Input: part model. Units: mm. Frame: model coordinates. Coordinates: 2 decimals unless noted, no trailing zeros. Order: outer loops, then holes, each group sorted by start corner. A loop starts at its lowest first (then second) coordinate and runs counter-clockwise, first axis right, second up. Notation, with made-up numbers: (-26, 75) - (-21, 75) arc R12 cw to (-21, 88) - close; hole circle Ø8 at (-11.75, 68). An arc over 180 degrees is marked (long way). Use a Markdown table: item, result. Add a question column.
from build123d import *

# Parameters (mm, degrees)
SKETCH1_R           = 9.486832981
BOSS_EXTRUDE1_DEPTH = 11
FILLET1_R           = 0.5


with BuildPart() as part:
    # Sketch1 → Boss-Extrude1 (new body)
    with BuildSketch(Plane(origin=(0, 0, 0), x_dir=(1, 0, 0), z_dir=(0, 1, 0))):
        with Locations(Location((0, 0, 0), (0, 0, 270))):
            Circle(SKETCH1_R)
    boss_extrude1 = extrude(amount=BOSS_EXTRUDE1_DEPTH)

    # Sketch2 → Revolve1 (revolve)
    with BuildSketch(Plane.XY):
        with BuildLine():
            Line((0, 24.281566173), (0, 11))
            Line((0, 11), (-15.178932769, 11))
            add(Edge.make_bspline(
                [(0, 24.281566173), (-13.015575695, 23.967255227), (-15.178932769, 11)],
                knots=[0, 0, 0, 1, 1, 1], degree=2))
        make_face()
    revolve1 = revolve(axis=Axis((0, 0, 0), (0, 1, 0)))

    # Mirror1: Boss-Extrude1, Revolve1 across plane
    add(boss_extrude1.mirror(Plane.ZX))
    add(revolve1.mirror(Plane.ZX))

    # Fillet1
    fillet1_edges = [part.edges().sort_by_distance(p)[0] for p in [
        (0, -11, -9.486832981),
        (0, 11, -9.486832981),
    ]]
    fillet(fillet1_edges, radius=FILLET1_R)


solid = part.part
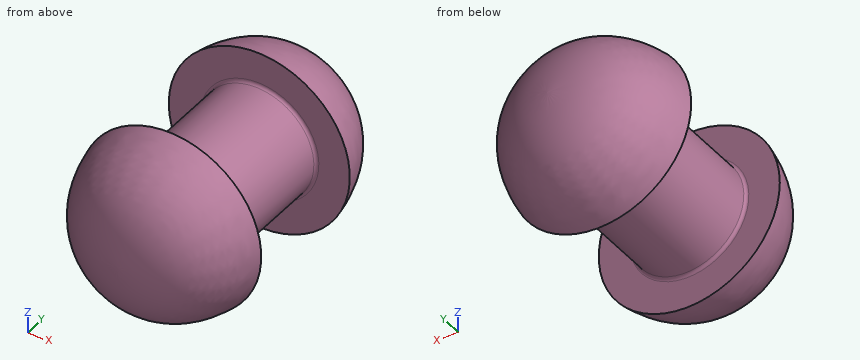
1) Cut plane A-A (y = -9). Return the cut outline in (x, z), and give its area (3 significant figures).
2) Contact query for flat-ended pins moving along their axis: P1, Ø4, axis at y = 17.5, z = -12, coming from the +X side; P2, Ø8, axis at x = 6.5, y = -8, coming from the -Z side; P3, Ø5, axis at x = -5, z = 1.5, coming from the +Y side. Output: stop coordinate, or through.
3) Material intervals for L1, parallel to Z at x = -0.5, y = 6.5; L2, parallel to Y at x = 3, z = 11; L3, parallel to Y at x = 9.5, z = -3, sorted ascending.
Computed:
| question | item | result |
|---|---|---|
| 1 | outline | circle Ø18.97 at (0, 0) |
| 1 | area | 283 mm2 |
| 2 | P1 | stops at x = 8.79 |
| 2 | P2 | stops at z = -14.68 |
| 2 | P3 | stops at y = 24.06 |
| 3 | L1 | z = -9.47 to 9.47 |
| 3 | L2 | y = -19.71 to -11, 11 to 19.71 |
| 3 | L3 | y = -21.09 to -11, 11 to 21.09 |
